Source: CAD feature listing. Evaluate the final solid. Frame: model axes, mm. Face numbers are marked on the shaded views. A direction names the side the tool comes from. Give positions to 0.01 mm unless a question says otherwise; leave off trailing zeros. Loops run counter-clockwise (first coordinate to the right, second up) from the corner with the lowest first, then second, coordinate; pieces in that order, holes last. Notation, with made-up numbers: (89.5, 42) -> (111.5, 42) arc R16 ccw to (111.5, 57) -> close; hole circle Ø11 at (24.25, 38). An arc over 180 degrees is marked (long way). Put each result on its own line as item: value.
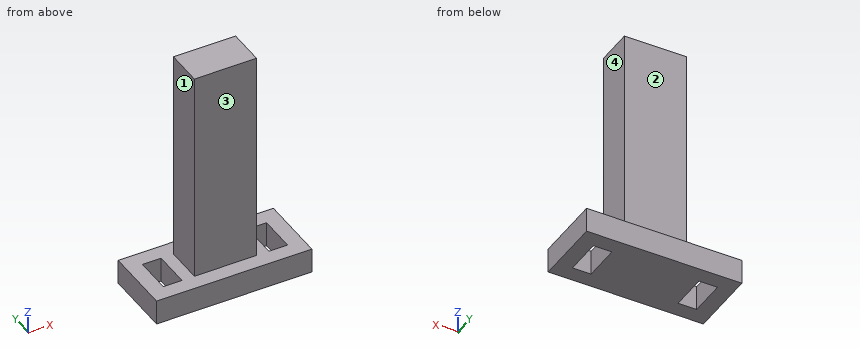
```python
from build123d import *

# Parameters (mm, degrees)
F0_W     = 15
F0_H     = 11
F1_DEPTH = 4
F2_W     = 10
F2_H     = 6
F3_DEPTH = 34.5
F0_W_2   = 5
F4_DEPTH = 4
F5_W     = 3
F5_H     = 6
F6_DEPTH = 4


with BuildPart() as f1:
    # F0 (on Top) → F1 (new body)
    with BuildSketch(Plane.XY):
        Rectangle(F0_W, F0_H)
    extrude(amount=F1_DEPTH)

    # F2 (on face) → F3 (join)
    with BuildSketch(Plane.XY.offset(4)):
        Rectangle(F2_W, F2_H)
    extrude(amount=F3_DEPTH)

    # F0 (on Top) → F4 (join)
    with BuildSketch(Plane.XY):
        Rectangle(F0_W, F0_H)
        with Locations((10, 0)):
            Rectangle(F0_W_2, F0_H)
        with Locations((-10, 0)):
            Rectangle(F0_W_2, F0_H)
    extrude(amount=F4_DEPTH)

    # F5 (on face) → F6 (cut)
    with BuildSketch(Plane.XY.offset(4)):
        with Locations((-8.5, 0)):
            Rectangle(F5_W, F5_H)
        with Locations((8.5, 0)):
            Rectangle(F5_W, F5_H)
    extrude(amount=-F6_DEPTH, mode=Mode.SUBTRACT)


solid = f1.part
```
(1) Section A-A on x = -8.75. Return loops of the section in (y, z), then the cut area to 3 significant figures.
Calculated:
outline: (-5.5, 0) -> (-3, 0) -> (-3, 4) -> (-5.5, 4) -> close; (3, 0) -> (5.5, 0) -> (5.5, 4) -> (3, 4) -> close
area: 20.0 mm²
(2) Line query: probe 1 along X at (y, z) = (2.25, 3.5); probe 2 along X at (y, z) = (0.25, 9.5); probe 3 along Y at (x, z) = (4, 36.5). Output: solid intervals per line, ascending. Write a range as from..to.
Calculated:
probe 1: x = -12.5..-10, -7..7, 10..12.5
probe 2: x = -5..5
probe 3: y = -3..3
(3) Section C-C on z = 31. Return loops of the section in (x, y), then the cut area to 3 significant figures.
Calculated:
outline: (-5, -3) -> (5, -3) -> (5, 3) -> (-5, 3) -> close
area: 60.0 mm²
(4) Section D-D on x = 3. Return loops of the section in (y, z), then the cut area to 3 significant figures.
Calculated:
outline: (-5.5, 0) -> (5.5, 0) -> (5.5, 4) -> (3, 4) -> (3, 38.5) -> (-3, 38.5) -> (-3, 4) -> (-5.5, 4) -> close
area: 251 mm²
(5) First-contact query: P1, Ø2, axis at y = -4.5, z = 17, coming from the +X side; P2, Ø6.5, axis at y = 1.5, z = 29.5, coming from the +X side; P3, Ø8, axis at x = -7.5, z = 17, coming from the +Y side; P4, Ø11, axis at x = -0.5, z = 16, coming from the -Y side. Flat tips, straight axial feed; report the tip coordinate or a pass-through.
Calculated:
P1: passes through
P2: stops at x = 5
P3: stops at y = 3
P4: stops at y = -3
(6) Section B-B on y = -0.25. Return loops of the section in (x, z).
Calculated:
outline: (-12.5, 0) -> (-10, 0) -> (-10, 4) -> (-12.5, 4) -> close; (-7, 0) -> (7, 0) -> (7, 4) -> (5, 4) -> (5, 38.5) -> (-5, 38.5) -> (-5, 4) -> (-7, 4) -> close; (10, 0) -> (12.5, 0) -> (12.5, 4) -> (10, 4) -> close
(7) Reachability of the marked faces 1, 2, 3 and 4 from +Z, -Z, +X, -X, +Y, -Y: full face, straight path, thin tool, end or side. Return the list, or none.
Calculated:
face 1: +Z, -X, +Y, -Y
face 2: +Z, +X, -X, +Y
face 3: +Z, +X, -X, -Y
face 4: +Z, +X, +Y, -Y
